Autodesk Inventor part; units mm, degrees
ref_plane "YZ Plane" through (0, 0, 0) normal (1, 0, 0) x (0, 1, 0)
ref_plane "XZ Plane" through (0, 0, 0) normal (0, 1, 0) x (-1, 0, 0)
ref_plane "XY Plane" through (0, 0, 0) normal (0, 0, 1) x (1, 0, 0)
sketch "草圖1" plane through (0, 0, 0) normal (0, 0, 1) x (1, 0, 0)
  line L0 (0, 0) -> (-50, 0) construction
  line L1 (0, 25) -> (-50, 25)
  line L2 (-50, -25) -> (0, -25)
  arc A0 (0, -25) -> (0, 25) centre (0, 0) ccw
  arc A1 (-50, 25) -> (-50, -25) centre (-50, 0) ccw
  line L3 (-25, 25) -> (-25, -25)
  point P0 (-25, 0)
  point P1 (25, 0)
  point P2 (-75, 0)
  dimension "d0" = 50
  dimension "d1" = 100
extrude "擠出1" add sketch "草圖1" along normal mid plane 3 contours L3 L2 A1 L1
sketch "草圖2" plane through (0, 0, 1.5) normal (0, 0, 1) x (1, 0, 0)
  arc A0 (-50, 25) -> (-50, -25) centre (-50, 0) ccw
  circle A1 centre (-50, 0) radius 25
  circle A2 centre (-50, 0) radius 22
  line L0 (-50, -25) -> (-25, -25)
  line L1 (-25, -25) -> (-25, 25)
  line L2 (-25, 25) -> (-50, 25)
  arc A3 (-50, 25) -> (-50, -25) centre (-50, 0) ccw
  point P0 (0, 0)
  point P1 (-50, 25)
  point P2 (-50, -25)
  dimension "d4" = 3
extrude "擠出2" add sketch "草圖2" against normal blind 41
sketch "草圖3" plane through (-25, -25, -1.5) normal (1, 0, 0) x (0, 0, 1)
  line L0 (-38, -50) -> (3, -50) construction
  line L1 (-38, -50) -> (-38, 0) construction
  line L2 (-38, 0) -> (3, 0) construction
  circle A0 centre (-17.5, -25) radius 1.5
  circle A1 centre (-27.5, -25) radius 1.5
  circle A2 centre (-17.5, -35) radius 1.5
  circle A3 centre (-7.5, -25) radius 1.5
  circle A4 centre (-17.5, -15) radius 1.5
  line L3 (-17.5, -50) -> (-17.5, 0) construction
  line L4 (3, 0) -> (3, -50)
  point P0 (1.5, -25)
  point P1 (-17.5, -25)
  dimension "d7" = 3
  dimension "d10" = 360
  dimension "d12" = 10
extrude "擠出3" cut sketch "草圖3" against normal up to surface
properties part number "Arm_5"
The listing builds one solid part. Answer for the finished solid, in the listing's coordinates (mm). A direction names the side the tool comes from. Round coordinates to 2 decimals unless told otherwise and drop trailing zeros. Order: outer loops, then holes, each group sorted by start corner. A loop starts at its lowest first (then second) coordinate and runs counter-clockwise, first axis right, second up. Notation, with made-up numbers: (-3, 57.5) - (19, 57.5) arc R13 ccw to (19, 68.5) - close; hole circle Ø2 at (77, 55.5). An arc over 180 degrees is marked (long way). Put each result on its own line as item: value. Start each with the question number.
(1) For faces 5 (the flat face through (-37, 25, -19)), 6 (the cylindrical face through (-29.68, -8.43, -20.23)), 7 (the cylindrical face through (-26.5, -0.07, -20.5)), determine the directions among +Z, -Z, +X, -X, +Y, -Y from which every point of the face is accessible in a straight line to the end or side of a thin tool.
(2) Find section A-A (y = -10). Give the vertices of the cut face in (x, z).
(3) Straight lines are drawn through the part: probe 1 along Y at (x, z) = (-26.9, -19); probe 2 along Z at (x, y) = (-27.35, 0); probe 3 along Z at (x, y) = (-29, -10). For each, find the intervals that lie inside material, in ascending order. Write a range as from..to.
(4) Find section B-B (z = -29). Give the vertices of the cut face in (x, y).
(5) Given P1, Ø5, axis at y = 0, z = -29, coming from the -X side; P2, Ø2, axis at y = 17, z = -27.5, coming from the -X side; P3, Ø3, axis at x = -50, y = 17, coming from the -Z side, each flat-ended and moving along its own axis, determine where each tip first touches the part or whether it passes through.
(6) Determine the mould class of faces 1 (the cylindrical face through (-26.5, -0.07, -10.5)), 2 (the flat face through (-50, 0, -1.5)), 3 (the flat face through (-38, -25, -19)), 4 (the cylindrical face through (-27.385, -11.487, -19.195)) for opening direction Z: released by +Z, released by -Z, zero draft, split by the parting line, or undercut.
(7) Find section C-C (x = -53). Give the vertices of the cut face in (y, z).
Reply:
1. face 5: +Z, -Z, +X, -X, +Y
1. face 6: -Z
1. face 7: +X
2. outline: (-72.91, -39.5) - (-69.6, -39.5) - (-69.6, -1.5) - (-30.4, -1.5) - (-30.4, -17.5) - (-25, -17.5) - (-25, 1.5) - (-72.91, 1.5) - close; (-30.4, -39.5) - (-25, -39.5) - (-25, -20.5) - (-30.4, -20.5) - close
3. probe 1: -25..-11.5, -8.5..-1.5, 1.5..8.5, 11.5..25
3. probe 2: -39.5..-30.5, -27.5..-20.5, -17.5..-10.5, -7.5..1.5
3. probe 3: -39.5..-20.5, -17.5..1.5
4. outline: (-50, -25) - (-25, -25) - (-25, -1.5) - (-28.05, -1.5) arc R22 cw (long way) to (-28.05, 1.5) - (-25, 1.5) - (-25, 25) - (-50, 25) arc R25 ccw to start
5. P1: x = -75
5. P2: x = -69.21
5. P3: z = -1.5
6. face 1: undercut
6. face 2: released by -Z
6. face 3: zero draft
6. face 4: undercut
7. outline: (-24.82, -39.5) - (-21.79, -39.5) - (-21.79, -1.5) - (21.79, -1.5) - (21.79, -39.5) - (24.82, -39.5) - (24.82, 1.5) - (-24.82, 1.5) - close
